CAD build for the part. Positions are in the model's coordinates, mm. Face numbers are marked on the shaded views. A direction names the side the tool comes from. Give positions to 0.01 mm unless a question says otherwise; leave off trailing zeros. Write each loop counter-clockwise with the first axis right and the second up, starting at its lowest first coordinate (ties: lowest second). Pieces come first, ordered by that corner, then holes. Notation, with made-up numbers: (33, 66) - (45, 66) arc R24 ccw to (45, 96) - close; hole circle Ø6 at (21.25, 0.5). An arc over 180 degrees is marked (long way). Put each result on its own line as item: value. Start each with the question number.
1. Drop flat-ended pins along their axis: pin 1 (0.5 mm diameter, centred on x = -12.5, y = 0, fed in from +Z); pin 2 (0.9 mm diameter, centred on y = 0, z = 11.5, fed in from -X); pin 3 (3 mm diameter, centred on y = -12.5, z = -0.5, fed in from +X); pin 4 (4.5 mm diameter, centred on x = 68.5, z = 0, fed in from -Y). Give the stop position or say it passes through.
2. Cut at A-A on x = 68.5. List the corners of the cut face in (y, z).
3. Wall check: line 1 (Z direction, x = 68.5, y = -27.95); line 2 (Y direction, x = -9, z = -5); line 3 (Z direction, x = 68, y = -28). Give the ranges that are in metal, low to high.
4. Tool access for the marked faces 1, 2 and 3: list every direction of +Z, -Z, +X, -X, +Y, -Y with a clear straight run to the whole face (end or side of a thin tool).
from build123d import *

# Parameters (mm, degrees)
F1_DEPTH = 16
F3_DEPTH = 12.5
F5_DEPTH = 12.5
F6_W     = 13
F6_H     = 7.5
F7_DEPTH = 12.5
F8_R     = 2.5
F9_DEPTH = 12.5
F10_R    = 0.2


with BuildPart() as f1:
    # F0 (on Top) → F1 (new body, symmetric)
    with BuildSketch(Plane.XY):
        with BuildLine():
            Line((-27.5, -1), (27.5, -1))
            ThreePointArc((27.5, -1), (48.3865985742, -9.0362658643), (58.5, -29))
            Line((58.5, -29), (76.5, -29))
            Line((76.5, -29), (76.5, -27))
            Line((76.5, -27), (60.2566787083, -27))
            ThreePointArc((60.2566787083, -27), (49.0464614264, -6.9539102055), (27.5, 1))
            Line((27.5, 1), (-27.5, 1))
            Line((-27.5, 1), (-27.5, -1))
        make_face()
    extrude(amount=F1_DEPTH, both=True)

    # F2 (on face) → F3 (cut, symmetric)
    with BuildSketch(Plane.XZ.offset(29)):
        with BuildLine():
            Line((76.5, 0), (76.5, 16))
            Line((76.5, 16), (73.5, 16))
            ThreePointArc((73.5, 16), (75.7435215896, 8.139410298), (76.5, 0))
        make_face()
        with BuildLine():
            Line((76.5, -16), (76.5, 0))
            ThreePointArc((76.5, 0), (75.7435215896, -8.139410298), (73.5, -16))
            Line((73.5, -16), (76.5, -16))
        make_face()
    extrude(amount=F3_DEPTH, both=True, mode=Mode.SUBTRACT)

    # F4 (on face) → F5 (cut, symmetric)
    with BuildSketch(Plane(origin=(0, 1, 0), x_dir=(-1, 0, 0), z_dir=(0, 1, 0))):
        with BuildLine():
            Line((27.5, -16), (27.5, -3.42e-08))
            ThreePointArc((27.5, -3.42e-08), (26.2208873777, -8.3815273234), (22.5, -16))
            Line((22.5, -16), (27.5, -16))
        make_face()
        with BuildLine():
            Line((27.5, -3.42e-08), (27.5, 16))
            Line((27.5, 16), (22.5, 16))
            ThreePointArc((22.5, 16), (26.2208873879, 8.3815272908), (27.5, -3.42e-08))
        make_face()
    extrude(amount=F5_DEPTH, both=True, mode=Mode.SUBTRACT)

    # F6 (on face) → F7 (cut, symmetric)
    with BuildSketch(Plane(origin=(0, 1, 0), x_dir=(-1, 0, 0), z_dir=(0, 1, 0))):
        with Locations((10, -12.25)):
            Rectangle(F6_W, F6_H)
        with Locations((10, 12.25)):
            Rectangle(F6_W, F6_H)
    extrude(amount=F7_DEPTH, both=True, mode=Mode.SUBTRACT)

    # F8 (on face) → F9 (cut, symmetric)
    with BuildSketch(Plane(origin=(0, -27, 0), x_dir=(-1, 0, 0), z_dir=(0, 1, 0))):
        with Locations((-68.5, 0)):
            Circle(F8_R)
    extrude(amount=F9_DEPTH, both=True, mode=Mode.SUBTRACT)

    # F10
    f10_edges = [f1.edges().sort_by_distance(p)[0] for p in [
        (76.5, -27, 0),
        (66.878339, -27, 16),
        (66.878339, -27, -16),
        (60.256679, -27, 0),
        (71, -27, 0),
        (49.046461, -6.95391, -16),
        (27.5, 1, 0),
        (49.046461, -6.95391, 16),
        (12, 1, 16),
        (-3.5, 1, 12.25),
        (-10, 1, 8.5),
        (-16.5, 1, 12.25),
        (-19.5, 1, 16),
        (-27.5, 1, 0),
        (-19.5, 1, -16),
        (-16.5, 1, -12.25),
        (-10, 1, -8.5),
        (-3.5, 1, -12.25),
        (12, 1, -16),
    ]]
    fillet(f10_edges, radius=F10_R)


solid = f1.part
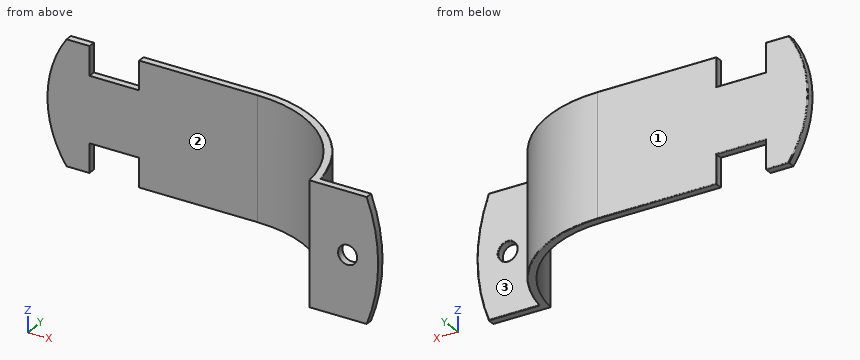
Report:
1. pin 1: stops at z = 8.5
1. pin 2: stops at x = -25.24
1. pin 3: stops at x = 55.25
1. pin 4: passes through
2. outline: (-29, -16) - (-27.2, -16) arc R0.2 ccw to (-27, -15.8) - (-27, -2.7) arc R0.2 ccw to (-27.2, -2.5) - (-29, -2.5) - close; (-29, 2.5) - (-27.2, 2.5) arc R0.2 ccw to (-27, 2.7) - (-27, 15.8) arc R0.2 ccw to (-27.2, 16) - (-29, 16) - close
3. line 1: z = -16 to -2.5, 2.5 to 16
3. line 2: y = -1 to 1
3. line 3: z = -16 to -2.45, 2.45 to 16
4. face 1: +Z, -Z, +X, -X, +Y
4. face 2: +Z, -Z, -X, -Y
4. face 3: +Z, -Z, +X, +Y
